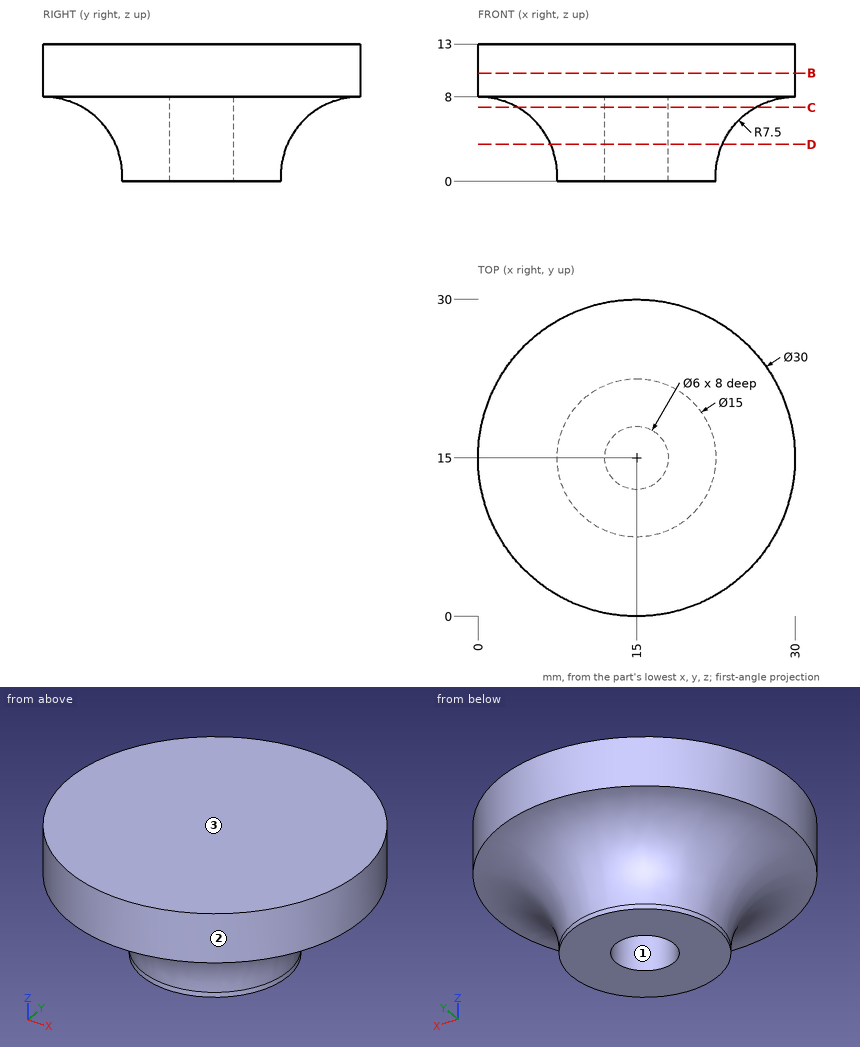
Check sheet for the drawn part. Datum: minimum x, y, z corner. Units: mm. Give positions to 0.01 mm unless a question says otherwise; leave off trailing zeros. Order: outer loops, then holes, each group sorted by start corner. A loop starts at its lowest first (then second) coordinate and runs counter-clockwise, first axis right, second up. Notation, with made-up numbers: (53.5, 89) - (74.5, 89) arc R12 cw to (74.5, 94) - close; hole circle Ø5 at (78.5, 75). An arc over 180 degrees is marked (long way). Answer as a JSON object with one key per item and string values.
(1) Material ranges on line 1 (X direction, y = 13, z = 2.5); line 2 (X direction, y = 15, z = 5.75); line 3 (Z direction, x = 2.5, y = 17.5), recorded low to high.
Report:
{"line 1": "7.49 to 12.76, 17.24 to 22.51", "line 2": "5.36 to 12, 18 to 24.64", "line 3": "7.65 to 13"}
(2) Draft check along Y on the marked faces 1, 2 and 3. Enter one of: released by +Y, released by -Y, zero draft, split by the parting line, or undercut.
Report:
{"face 1": "undercut", "face 2": "split by the parting line", "face 3": "zero draft"}
(3) Cross-section at C-C (z = 7). Record the cut outline in (x, y), then the cut area to 3 significant figures.
Report:
{"outline": "circle Ø22.52 at (15, 15); hole circle Ø6 at (15, 15)", "area": "370 mm^2"}
(4) Cross-section at B-B (z = 10.25). Record the cut outline in (x, y), then the cut area to 3 significant figures.
Report:
{"outline": "circle Ø30 at (15, 15)", "area": "707 mm^2"}
(5) Cross-section at D-D (z = 3.5). Record the cut outline in (x, y).
Report:
{"outline": "circle Ø16.25 at (15, 15); hole circle Ø6 at (15, 15)"}
(6) Depth check by flat-ended pin: pin 1 Ø3 at (y, z) = (14, 5) entering from -X; pin 2 Ø6 at (x, z) = (5.5, 8.5) entering from -Y. Enter the tip coordinate at first touch or a pass-through.
Report:
{"pin 1": "x = 4.54", "pin 2": "y = 1.48"}
